from build123d import *

# Parameters (mm, degrees)
EXTRUDE_1_DEPTH     = 10
EXTRUDE_2_DEPTH     = 10
EXTRUDE_START       = 200
EXTRUDE_3_DEPTH     = 200
CUT_EXTRUDE_1_DEPTH = 294.811163845


with BuildPart() as part:
    # 草图1 → 凸台-拉伸1 (new body)
    with BuildSketch(Plane(origin=(0, 0, 0), x_dir=(1, 0, 0), z_dir=(0, 1, 0))):
        with BuildLine():
            Line((-75, 95), (75, 95))
            ThreePointArc((75, 95), (170, 0), (75, -95))
            Line((75, -95), (-75, -95))
            ThreePointArc((-75, -95), (-170, 0), (-75, 95))
        make_face()
    extrude(amount=EXTRUDE_1_DEPTH)

    # 草图2 → 凸台-拉伸2 (add)
    with BuildSketch(Plane(origin=(0, 10, 0), x_dir=(1, 0, 0), z_dir=(0, 1, 0))):
        with BuildLine():
            Line((-75, 85), (75, 85))
            ThreePointArc((75, 85), (160, 0), (75, -85))
            Line((75, -85), (-75, -85))
            ThreePointArc((-75, -85), (-160, 0), (-75, 85))
        make_face()
    extrude(amount=EXTRUDE_2_DEPTH)

    # 草图3 → 凸台-拉伸3 (add)
    with BuildSketch(Plane.XZ.offset(EXTRUDE_START)):
        with BuildLine():
            Line((-75, -85), (75, -85))
            ThreePointArc((75, -85), (160, 0), (75, 85))
            Line((75, 85), (-75, 85))
            ThreePointArc((-75, 85), (-160, 0), (-75, -85))
        make_face()
    extrude(amount=-EXTRUDE_3_DEPTH)

    # 草图4 → 切除-拉伸1 (cut, through all)
    with BuildSketch(Plane(origin=(0, 20, 0), x_dir=(1, 0, 0), z_dir=(0, 1, 0))):
        with BuildLine():
            Line((-75, 75), (75, 75))
            ThreePointArc((75, 75), (150, 0), (75, -75))
            Line((75, -75), (-75, -75))
            ThreePointArc((-75, -75), (-150, 0), (-75, 75))
        make_face()
    extrude(amount=-CUT_EXTRUDE_1_DEPTH, mode=Mode.SUBTRACT)


solid = part.part
Model file for the job. Use its own axes, mm. A direction names the side the tool comes from. Give positions to 0.01 mm unless a question says otherwise; leave off trailing zeros. Write each loop counter-clockwise with the first axis right and the second up, starting at its lowest first coordinate (ties: lowest second). Pieces come first, ordered by that corner, then holes. Notation, with made-up numbers: M 59.25,80.25 L 97.25,80.25 A10 ccw 97.25,91.25 Z; hole C -17.5,-30.75 d11. An arc over 180 degrees is marked long. One line per item, written item: value. Start each with the question number.
Q1. Two-plate mould, pull along Z, no slides. Class faces 4 (the cylindrical face through (159.98, 14.93, -1.87)), 5 (the flat face through (1, -88, 75)), 6 (the flat face through (-13, -200, 76)): +Z half, -Z half, draft (parallel to the pull), parting line (faces both ways), or undercut.
Q2. Saw through at B-B, the plane x = -31.5. Write the cut outline in (y, z).
Q3. Drop flat-ended pins along their axis: pin 1 Ø1.5 at (x, y) = (-23.5, -10) entering from -Z; pin 2 Ø4 at (x, y) = (113, -48.5) entering from -Z; pin 3 Ø10 at (y, z) = (-39.5, 10) entering from +X. Give the stop position or say it passes through.
Q4. Saw through at C-C, the plane y = -144. Write the cut outline in (x, z).
Q5. 3-axis set-ups, long thin cutter, end or side, ignore diameter. For faces 1 (the flat face through (-1, 15, -85)), 2 (the cylindrical face through (149.98, -88.46, -1.65)), 3 (the flat face through (1, 15, 85)): which of +Z, -Z, +X, -X, +Y, -Y reach the whole face in a straight line?
Q6. Saw through at A-A, the plane z = 0. Write the cut outline in (x, y), plus the area to 3 significant figures.
Q7. Probe probe 1 along Z at (x, y) = (75, -34); probe 2 along X at (y, z) = (-18.5, -2); probe 3 along X at (y, z) = (-154, 65). List the from-to ranges inside material, lowest first. Write a range as [from, to].
Output values:
1. face 4: parting line
1. face 5: undercut
1. face 6: draft
2. outline: M -200,-85 L 0,-85 L 0,-95 L 10,-95 L 10,-85 L 20,-85 L 20,-75 L -200,-75 Z; M -200,75 L 20,75 L 20,85 L 10,85 L 10,95 L 0,95 L 0,85 L -200,85 Z
3. pin 1: stops at z = -85
3. pin 2: stops at z = -77
3. pin 3: stops at x = 159.85
4. outline: M -75,-85 L 75,-85 A85 ccw 75,85 L -75,85 A85 ccw Z; hole M -75,-75 L 75,-75 A75 ccw 75,75 L -75,75 A75 ccw Z
5. face 1: -Z, +X, -X, +Y
5. face 2: +Y, -Y
5. face 3: +Z, +X, -X, +Y
6. outline: M -170,0 L -160,0 L -160,-200 L -150,-200 L -150,20 L -160,20 L -160,10 L -170,10 Z; M 150,-200 L 160,-200 L 160,0 L 170,0 L 170,10 L 160,10 L 160,20 L 150,20 Z
6. area: 4,600 mm²
7. probe 1: z = [-85, -75], [75, 85]
7. probe 2: x = [-159.98, -149.97], [149.97, 159.98]
7. probe 3: x = [-129.77, -112.42], [112.42, 129.77]
